Autodesk Inventor part; units mm, degrees
ref_plane "YZ Plane" through (0, 0, 0) normal (1, 0, 0) x (0, 1, 0)
ref_plane "XZ Plane" through (0, 0, 0) normal (0, 1, 0) x (-1, 0, 0)
ref_plane "XY Plane" through (0, 0, 0) normal (0, 0, 1) x (1, 0, 0)
sketch "Sketch1" plane through (0, 0, 0) normal (0, 0, 1) x (1, 0, 0)
  arc A0 (-1.5875, 55.2682) -> (1.5875, 55.2682) centre (0, 0) ccw
  circle A1 centre (0, 0) radius 50.8
  line L0 (0, 79.3124) -> (0, -77.7249) construction
  line L1 (-77.4074, 0) -> (77.4074, 0) construction
  circle A2 centre (0, 0) radius 52.8955 construction
  circle A3 centre (-1.846, 52.8633) radius 0.75
  circle A4 centre (1.846, 52.8633) radius 0.75
  circle A5 centre (-52.8633, -1.846) radius 0.75
  circle A6 centre (-52.8633, 1.846) radius 0.75
  circle A7 centre (1.846, -52.8633) radius 0.75
  circle A8 centre (-1.846, -52.8633) radius 0.75
  circle A9 centre (52.8633, 1.846) radius 0.75
  circle A10 centre (52.8633, -1.846) radius 0.75
  arc A11 (1.5875, 55.291) -> (-1.5875, 55.291) centre (0, 55.291) ccw
  line L2 (-1.5875, 55.291) -> (-1.5875, 55.2682)
  line L3 (1.5875, 55.291) -> (1.5875, 55.2682)
  dimension "d0" = 110.582
  dimension "d1" = 101.6
  dimension "d4" = 105.791
  dimension "d5" = 4
  dimension "d6" = 1.5
  dimension "d9" = 360
  dimension "d11" = 3.175
extrude "Extrusion1" add sketch "Sketch1" against normal blind 1.5
properties part number "J005536" material "ACRYLIC, CLEAR"
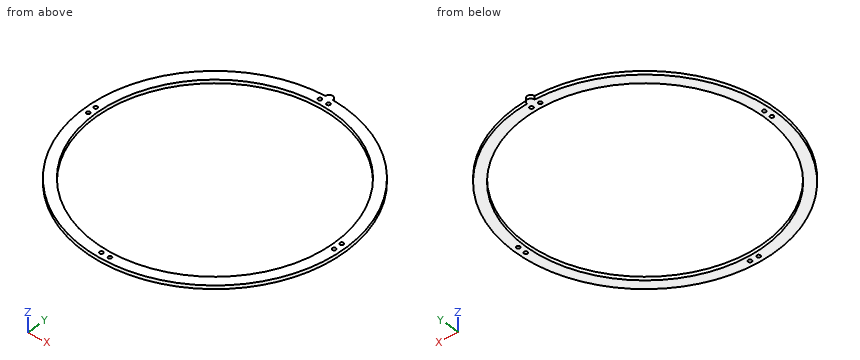
Geometry check sheet. Reference: the model listing, model coordinates, mm. Round coordinates to 2 decimals unless told otherwise and drop trailing zeros. Loops run counter-clockwise (first coordinate to the right, second up) from the corner with the lowest first, then second, coordinate; pieces in that order, holes last.
Item 1: Cross-section at A-A on x = 45.5. Record the boundary of the cut face in (y, z).
Item 2: Gauge pin test, flat end, axial feed: pin 1 (1.4 mm diameter, centred on x = -1.85, y = -52.86, fed in from +Z). Record the tip position at first contact, or that the pin passes through.
Item 3: Cross-section at C-C on z = -0.6. Count the separate pieces of the cut face and the enclosed holes in it, then the cut area to 3 significant figures.
Item 4: Thickness scan on line 1 (Y direction, x = 16.5, z = -0.35); line 2 (X direction, y = 3.5, z = -1.3); line 3 (Y direction, x = 2.5, z = -0.1). Record the ranges inside material, lowest first.
Item 5: Cross-section at B-B on y = -22.5. Record the boundary of the cut face in (x, z).
Answer sheet:
1. outline: (-31.41, -1.5) - (-22.59, -1.5) - (-22.59, 0) - (-31.41, 0) - close; (22.59, -1.5) - (31.41, -1.5) - (31.41, 0) - (22.59, 0) - close
2. pin 1: passes through
3. separate pieces: 1
3. enclosed holes: 9
3. area: 1,490 mm2
4. line 1: y = -52.77 to -48.05, 48.05 to 52.77
4. line 2: x = -55.18 to -50.68, 50.68 to 55.18
4. line 3: y = -55.23 to -53.23, -52.5 to -50.74, 50.74 to 52.5, 53.23 to 55.23
5. outline: (-50.51, -1.5) - (-45.55, -1.5) - (-45.55, 0) - (-50.51, 0) - close; (45.55, -1.5) - (50.51, -1.5) - (50.51, 0) - (45.55, 0) - close
